Autodesk Inventor part; units mm, degrees
ref_plane "YZ Plane" through (0, 0, 0) normal (1, 0, 0) x (0, 1, 0)
ref_plane "XZ Plane" through (0, 0, 0) normal (0, 1, 0) x (-1, 0, 0)
ref_plane "XY Plane" through (0, 0, 0) normal (0, 0, 1) x (1, 0, 0)
sketch "Sketch1" plane through (0, 0, 0) normal (0, 1, 0) x (-1, 0, 0)
  circle A0 centre (0, 0) radius 0.7
  dimension "d0" = 1.4
extrude "Extrusion1" add sketch "Sketch1" along normal blind 10
thread "Thread1"
sketch "Sketch2" plane through (0, 10, 0) normal (0, 1, 0) x (1, 0, 0)
  circle A0 centre (0, 0) radius 1.25
  dimension "d5" = 2.5
extrude "Extrusion2" add sketch "Sketch2" along normal blind 0.8
fillet "Fillet1" radius 0.2 1 edges at (-1.25, 10.8, 0)
properties part number "m1_4_10mm_screw"
Work out the finished part from the listing and answer in its coordinate system (mm). A direction names the side the tool comes from. Give positions to 0.01 mm unless a question says otherwise; leave off trailing zeros. Write each loop counter-clockwise with the first axis right and the second up, starting at its lowest first coordinate (ties: lowest second). Pieces come first, ordered by that corner, then holes. Notation, with made-up numbers: (85.5, 48) - (99.5, 48) arc R28 cw to (99.5, 77) - close; hole circle Ø8 at (55.5, 43). An arc over 180 degrees is marked (long way). Use one line per item in the form item = value.
1. Consider L1, parallel to Y at x = -0.05, z = -0.95; L2, parallel to Z at x = 0, y = 3; L3, parallel to Z at x = 0.4, y = 1.25. Determine where each line is inside the solid, lowest interval first.
Filled in:
L1 = 10 to 10.8
L2 = -0.7 to 0.7
L3 = -0.57 to 0.57
2. A cutting plane is placed at B-B (z = 0). Write down the section's boundary in (x, y), and give its area (3 significant figures).
Filled in:
outline = (-1.25, 10) - (-0.7, 10) - (-0.7, 0) - (0.7, 0) - (0.7, 10) - (1.25, 10) - (1.25, 10.6) arc R0.2 ccw to (1.05, 10.8) - (-1.05, 10.8) arc R0.2 ccw to (-1.25, 10.6) - close
area = 16.0 mm^2
3. A cutting plane is placed at A-A (x = 0). Write down the section's boundary in (y, z).
Filled in:
outline = (0, -0.7) - (10, -0.7) - (10, -1.25) - (10.6, -1.25) arc R0.2 ccw to (10.8, -1.05) - (10.8, 1.05) arc R0.2 ccw to (10.6, 1.25) - (10, 1.25) - (10, 0.7) - (0, 0.7) - close
4. A cutting plane is placed at C-C (y = 8.25). Write down the section's boundary in (x, z), and give its area (3 significant figures).
Filled in:
outline = circle Ø1.4 at (0, 0)
area = 1.54 mm^2
5. For faces 1 (the face through (1, 10, 0)), 2 (the face through (-0.27, 10.3, -1.22)), determine the directions among +Z, -Z, +X, -X, +Y, -Y from which every point of the face is accessible in a straight line to the end or side of a thin tool.
Filled in:
face_1 = -Y
face_2 = +Y, -Y
